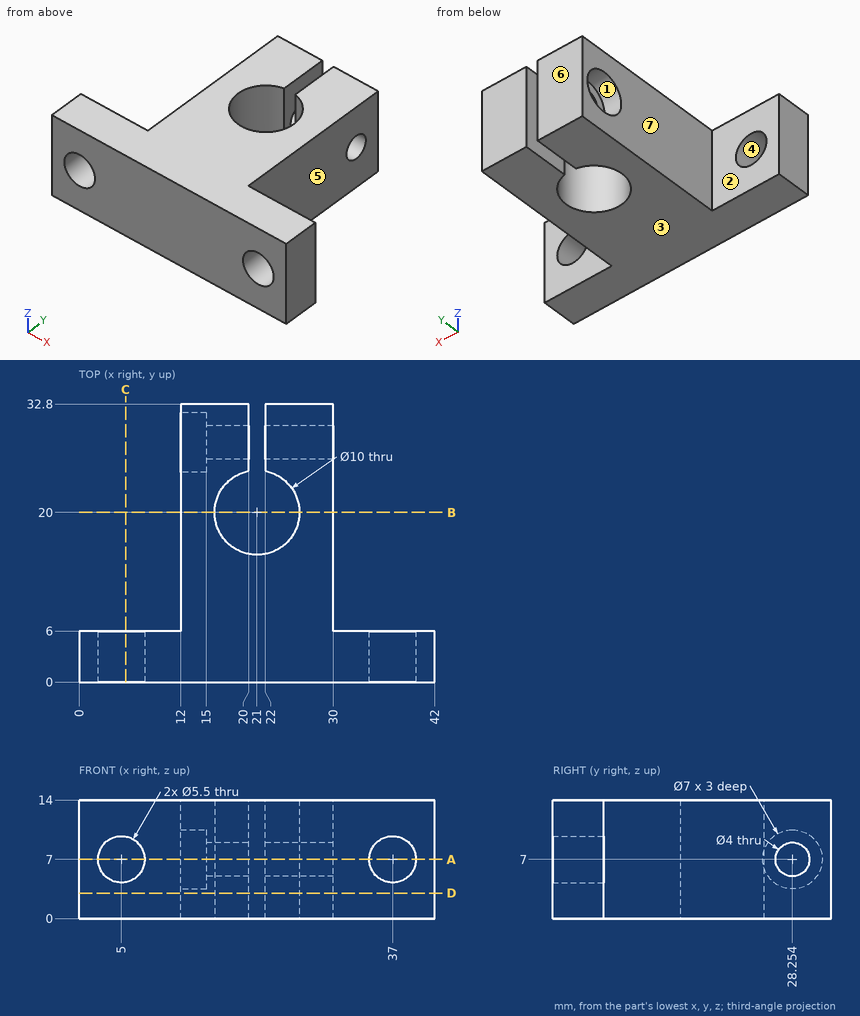
Geometry: see drawing. Coordinates: mm, zero at the bounding-box minimum. A direction names the side the tool comes from. Give positions to 0.01 mm unless a question says otherwise; leave off trailing zeros. Write each loop counter-clockwise with the first axis right and the second up, starting at its lowest first coordinate (ties: lowest second). Pieces come first, ordered by that corner, then holes. Notation, with made-up numbers: M 0,9 L 49,9 A20 ccw 49,28 Z; hole C 73.5,25.25 d10. An arc over 180 degrees is marked long. Answer in a Markdown table with one row per item. Add a question column.
(1) Reachability of the marked faces 5, 6 and 7 from +Z, -Z, +X, -X, +Y, -Y: full face, straight path, thin tool, end or side. Return the list, or none.
(2) Section C-C on x = 5.5. Return loops of the section in (y, z).
(3) First-contact query: pin 1 (4 mm diameter, centred on y = 28, z = 5, fed in from +X); pin 2 (4 mm diameter, centred on y = 24.5, z = 9, fed in from -X); pin 3 (6 mm diameter, centred on x = 39, z = 7.5, fed in from +Y); pin 4 (8 mm diameter, centred on x = 21, y = 20, fed in from +Z). Flat tips, straight axial feed; report the tip coordinate or a pass-through.
(4) Ray query, line 1 (X direction, y = 1.4, z = 7); line 2 (X direction, y = 28.5, z = 11.5); line 3 (Y direction, x = 17.05, z = 7) (1 decimal). Return the intervals inside material, ascending.
(5) Section D-D on z = 3. Return loops of the section in (x, y).
(6) Section A-A on z = 7. State how many separate pieces and enclosed holes the cut face has, and give its area (3 significant figures).
(7) Mould query, pull axis Z, two halves, no side actions, for the marked faces 1, 2, 3 and 4. Classes: +Z half, -Z half, draft (parallel to the pull), parting line (faces both ways), or undercut.
(8) Section B-B on y = 20. Return loops of the section in (x, z), and give its area (3 significant figures).
Result set:
| question | item | result |
|---|---|---|
| 1 | face 5 | +Z, -Z, +X, +Y |
| 1 | face 6 | +Z, -Z, +X, -X, +Y |
| 1 | face 7 | +Z, -Z, -X, +Y |
| 2 | outline | M 0,0 L 6,0 L 6,4.3 L 0,4.3 Z; M 0,9.7 L 6,9.7 L 6,14 L 0,14 Z |
| 3 | pin 1 | stops at x = 30 |
| 3 | pin 2 | stops at x = 12 |
| 3 | pin 3 | stops at y = 6 |
| 3 | pin 4 | passes through |
| 4 | line 1 | x = 0 to 2.25, 7.75 to 34.25, 39.75 to 42 |
| 4 | line 2 | x = 12 to 20, 22 to 30 |
| 4 | line 3 | y = 0 to 16.9, 23.1 to 26.3, 30.3 to 32.8 |
| 5 | outline | M 0,0 L 42,0 L 42,6 L 30,6 L 30,32.8 L 22,32.8 L 22,24.9 A5 cw long 20,24.9 L 20,32.8 L 12,32.8 L 12,6 L 0,6 Z |
| 6 | separate pieces | 5 |
| 6 | enclosed holes | 0 |
| 6 | area | 501 mm^2 |
| 7 | face 1 | undercut |
| 7 | face 2 | draft |
| 7 | face 3 | -Z half |
| 7 | face 4 | undercut |
| 8 | outline | M 12,0 L 16,0 L 16,14 L 12,14 Z; M 26,0 L 30,0 L 30,14 L 26,14 Z |
| 8 | area | 112 mm^2 |
